```python
from build123d import *

# Parameters (mm, degrees)
SKETCH1_W           = 431.8
SKETCH1_H           = 95.25
BOSS_EXTRUDE1_DEPTH = 6.35
SKETCH2_W           = 12.7
SKETCH2_H           = 6.35
CUT_EXTRUDE1_DEPTH  = 7.35
LPATTERN1_COUNT     = 17
LPATTERN1_PITCH     = 25.4
SKETCH3_W           = 6.35
SKETCH3_H           = 6.35
CUT_EXTRUDE2_DEPTH  = 7.35
SKETCH5_W           = 6.35
SKETCH5_H           = 12.7
CUT_EXTRUDE4_DEPTH  = 7.35
LPATTERN2_COUNT     = 2
LPATTERN2_PITCH     = 25.4
LPATTERN2_COL_COUNT = 2
LPATTERN2_COL_PITCH = 25.4
SKETCH6_W           = 114.3
SKETCH6_H           = 46.0375
CUT_EXTRUDE5_DEPTH  = 7.35
SKETCH7_R           = 1.75
CUT_EXTRUDE6_DEPTH  = 7.35
SKETCH8_W           = 6.35
SKETCH8_H           = 9.525
SKETCH8_H_2         = 12.7
CUT_EXTRUDE7_DEPTH  = 7.35
LPATTERN3_COUNT     = 2
LPATTERN3_PITCH     = 425.45


with BuildPart() as part:
    # Sketch1 → Boss-Extrude1 (new body)
    with BuildSketch(Plane(origin=(0, 0, 0), x_dir=(1, 0, 0), z_dir=(0, 1, 0))):
        with Locations((215.9, 47.625)):
            Rectangle(SKETCH1_W, SKETCH1_H)
    extrude(amount=BOSS_EXTRUDE1_DEPTH)

    # Sketch2 → Cut-Extrude1 (cut, through all)
    with BuildSketch(Plane(origin=(0, 6.35, 0), x_dir=(1, 0, 0), z_dir=(0, 1, 0))):
        with Locations((12.7, 92.075)):
            Rectangle(SKETCH2_W, SKETCH2_H)
        with Locations((12.7, 3.175)):
            Rectangle(SKETCH2_W, SKETCH2_H)
    cut_extrude1 = extrude(amount=-CUT_EXTRUDE1_DEPTH, mode=Mode.SUBTRACT)

    # LPattern1: Cut-Extrude1 ×17
    with Locations(*[(i * LPATTERN1_PITCH, 0, 0) for i in range(1, LPATTERN1_COUNT)]):
        add(cut_extrude1, mode=Mode.SUBTRACT)

    # Sketch3 → Cut-Extrude2 (cut, through all)
    with BuildSketch(Plane(origin=(0, 6.35, 0), x_dir=(1, 0, 0), z_dir=(0, 1, 0))):
        with Locations((3.175, 92.075)):
            Rectangle(SKETCH3_W, SKETCH3_H)
        with Locations((3.175, 3.175)):
            Rectangle(SKETCH3_W, SKETCH3_H)
        with Locations((428.625, 92.075)):
            Rectangle(SKETCH3_W, SKETCH3_H)
        with Locations((428.625, 3.175)):
            Rectangle(SKETCH3_W, SKETCH3_H)
    extrude(amount=-CUT_EXTRUDE2_DEPTH, mode=Mode.SUBTRACT)

    # Sketch5 → Cut-Extrude4 (cut, through all)
    with BuildSketch(Plane(origin=(0, 6.35, 0), x_dir=(1, 0, 0), z_dir=(0, 1, 0))):
        with Locations((187.325, 47.625)):
            Rectangle(SKETCH5_W, SKETCH5_H)
        with Locations((307.975, 47.625)):
            Rectangle(SKETCH5_W, SKETCH5_H)
    cut_extrude4 = extrude(amount=-CUT_EXTRUDE4_DEPTH, mode=Mode.SUBTRACT)

    # LPattern2: Cut-Extrude4 ×2
    with Locations(*[(0, 0, -i * LPATTERN2_PITCH) for i in range(1, LPATTERN2_COUNT)]):
        add(cut_extrude4, mode=Mode.SUBTRACT)

    # LPattern2 col: Cut-Extrude4 ×2
    with Locations(*[(0, 0, i * LPATTERN2_COL_PITCH) for i in range(1, LPATTERN2_COL_COUNT)]):
        add(cut_extrude4, mode=Mode.SUBTRACT)

    # Sketch6 → Cut-Extrude5 (cut, through all)
    with BuildSketch(Plane(origin=(0, 6.35, 0), x_dir=(1, 0, 0), z_dir=(0, 1, 0))):
        with Locations((247.65, 47.625)):
            Rectangle(SKETCH6_W, SKETCH6_H)
    extrude(amount=-CUT_EXTRUDE5_DEPTH, mode=Mode.SUBTRACT)

    # Sketch7 → Cut-Extrude6 (cut, through all)
    with BuildSketch(Plane(origin=(0, 6.35, 0), x_dir=(1, 0, 0), z_dir=(0, 1, 0))):
        with Locations((52.65, 44.45)):
            Circle(SKETCH7_R)
        with Locations((116.65, 44.45)):
            Circle(SKETCH7_R)
        with Locations((315.15, 44.45)):
            Circle(SKETCH7_R)
        with Locations((379.15, 44.45)):
            Circle(SKETCH7_R)
    extrude(amount=-CUT_EXTRUDE6_DEPTH, mode=Mode.SUBTRACT)

    # Sketch8 → Cut-Extrude7 (cut, through all)
    with BuildSketch(Plane(origin=(0, 6.35, 0), x_dir=(1, 0, 0), z_dir=(0, 1, 0))):
        with Locations((3.175, 84.1375)):
            Rectangle(SKETCH8_W, SKETCH8_H)
        with Locations((3.175, 11.1125)):
            Rectangle(SKETCH8_W, SKETCH8_H)
        with Locations((3.175, 34.925)):
            Rectangle(SKETCH8_W, SKETCH8_H_2)
        with Locations((3.175, 60.325)):
            Rectangle(SKETCH8_W, SKETCH8_H_2)
    cut_extrude7 = extrude(amount=-CUT_EXTRUDE7_DEPTH, mode=Mode.SUBTRACT)

    # LPattern3: Cut-Extrude7 ×2
    with Locations(*[(i * LPATTERN3_PITCH, 0, 0) for i in range(1, LPATTERN3_COUNT)]):
        add(cut_extrude7, mode=Mode.SUBTRACT)


solid = part.part
```
Part model, mm, in its own coordinate system. Coordinates: 2 decimals unless noted, no trailing zeros. Order: outer loops, then holes, each group sorted by start corner. A loop starts at its lowest first (then second) coordinate and runs counter-clockwise, first axis right, second up. Notation, with made-up numbers: (4.25, 54) - (40.25, 54) arc R11 ccw to (40.25, 73) - close; hole circle Ø6 at (-5.5, 83.5). An arc over 180 degrees is marked (long way). Return JSON: item names as keys, results as strings. Group by question number.
Item 1: Cut at A-A (z = -20). List the corners of the cut face in (x, y).
Item 2: Drill centre lines: probe 1 along X at (y, z) = (3.25, -44.45); probe 2 along X at (y, z) = (5, -74); probe 3 along Z at (x, y) = (238, 3). Where is each one in solid material? Low to high. Write a range as from..to.
Item 3: Cut at C-C (z = -63). List the corners of the cut face in (x, y), plus the area to 3 significant figures.
Item 4: Pin check, flat tips, straight feed: pin 1 (3 mm diameter, centred on x = 430, y = 2, fed in from -Z) (3 decimals); pin 2 (1.9 mm diameter, centred on x = 188, y = 2, fed in from +Z); pin 3 (1.9 mm diameter, centred on y = 1.5, z = -10, fed in from +X). Stop position of each tip, or through.
Item 5: Cut at B-B (x = 280). List the corners of the cut face in (y, z), plus the area to 4 significant figures.
Item 6: Cut at D-D (y = 2). State how many separate pieces and enclosed holes the cut face has, plus the area to 3 significant figures.
Check values:
{
 "1": {"outline": "(0, 0) - (184.15, 0) - (184.15, 6.35) - (0, 6.35) - close; (190.5, 0) - (304.8, 0) - (304.8, 6.35) - (190.5, 6.35) - close; (311.15, 0) - (431.8, 0) - (431.8, 6.35) - (311.15, 6.35) - close"},
 "2": {"probe 1": "x = 0..50.9, 54.4..114.9, 118.4..184.15, 311.15..313.4, 316.9..377.4, 380.9..431.8", "probe 2": "x = 0..184.15, 190.5..304.8, 311.15..431.8", "probe 3": "z = -88.9..-70.64, -24.61..-6.35"},
 "3": {"outline": "(6.35, 0) - (190.5, 0) - (190.5, 6.35) - (6.35, 6.35) - close; (304.8, 0) - (425.45, 0) - (425.45, 6.35) - (304.8, 6.35) - close", "area": "1,940 mm2"},
 "4": {"pin 1": "stops at z = -79.375", "pin 2": "stops at z = -6.35", "pin 3": "stops at x = 425.45"},
 "5": {"outline": "(0, -95.25) - (6.35, -95.25) - (6.35, -70.64) - (0, -70.64) - close; (0, -24.61) - (6.35, -24.61) - (6.35, 0) - (0, 0) - close", "area": "312.5 mm2"},
 "6": {"separate pieces": "1", "enclosed holes": "5", "area": "31,900 mm2"}
}
